Part model, mm, in its own coordinate system. A direction names the side the tool comes from. Coordinates: 2 decimals unless noted, no trailing zeros. Write each loop counter-clockwise with the first axis right and the second up, starting at its lowest first coordinate (ties: lowest second). Pieces come first, ordered by that corner, then holes. Notation, with made-up numbers: (89.25, 12.5) -> (111.25, 12.5) arc R22 cw to (111.25, 47.5) -> close; hole circle Ø11 at (87.25, 13.5). An arc over 180 degrees is marked (long way). Write item = value, one per line. Start each with the question number.
Q1. Band-saw the part on C-C, the plane y = -10.5. List the corners of the cut face in (x, z), plus the area to 3 significant figures.
Q2. Pull direction Z, two halves, no side cores. Call faces 5 (the flat face through (-13, 3, 15.47)), 6 (the flat face through (0, 1, 3)), 7 (the flat face through (-13, 3, 25.4)): released by +Z, released by -Z, zero draft, split by the parting line, or undercut.
Q3. Band-saw the part on D-D, the plane x = -13. List the corners of the cut face in (y, z), plus the area to 3 significant figures.
Q4. Pin check, flat tips, straight feed: P1, Ø5, axis at x = -8, y = -6.5, coming from the +Z side; P2, Ø5, axis at x = -7, z = 3.5, coming from the -Y side. Stop position of each tip, or through.
Q5. Tool access for faces 1 (the flat face through (-20.222, -13, -3)), 2 (the flat face through (-9.744, 3, 12)), 3 (the flat face through (-13, 0, 16)), 4 (the flat face through (-13, 6.35, 6)): list every direction of +Z, -Z, +X, -X, +Y, -Y with a clear straight run to the whole face (end or side of a thin tool).
Q6. Probe line 1 (Z direction, x = -15, y = 1.5); line 2 (Y direction, x = -6.25, z = -5); line 3 (Z direction, x = -3.75, y = -10). List the from-to ranges inside material, lowest first.
Q7. Band-saw the part on B-B, the plane z = 11. List the corners of the cut face in (x, y).
Q8. Band-saw the part on A-A, the plane x = -18.5. List the corners of the cut face in (y, z), plus the area to 3 significant figures.
Autodesk Inventor part; units mm, degrees
ref_plane "YZ Plane" through (0, 0, 0) normal (1, 0, 0) x (0, 1, 0)
ref_plane "XZ Plane" through (0, 0, 0) normal (0, 1, 0) x (-1, 0, 0)
ref_plane "XY Plane" through (0, 0, 0) normal (0, 0, 1) x (1, 0, 0)
sketch "Sketch1" plane through (0, 0, 0) normal (0, 1, 0) x (-1, 0, 0)
  line L0 (0, 0) -> (25.4, 0)
  line L1 (25.4, 0) -> (25.4, 25.4)
  line L2 (25.4, 25.4) -> (0, 25.4)
  line L3 (0, 25.4) -> (0, 0)
  dimension "d0" = 25.4
  dimension "d1" = 25.4
extrude "Extrusion1" add sketch "Sketch1" along normal blind 6.35
sketch "Sketch2" plane through (0, 6.35, 0) normal (0, 1, 0) x (1, 0, 0)
  line L0 (0, 0) -> (-25.4, 0)
  line L1 (0, 0) -> (-25.4, 0)
  line L2 (-25.4, 0) -> (-25.4, 6.35)
  line L3 (-25.4, 6.35) -> (0, 6.35)
  line L4 (0, 6.35) -> (0, 0)
  dimension "d4" = 6.35
extrude "Extrusion2" add sketch "Sketch2" against normal blind 31.75
sketch "Sketch3" plane through (-25.4, 0, 0) normal (0, 0, 1) x (1, 0, 0)
  line L0 (5.1775, -6.7435) -> (19.8333, -6.7435)
  line L1 (19.8333, -6.7435) -> (19.8333, -19.4435)
  line L2 (19.8333, -19.4435) -> (5.1775, -19.4435)
  line L3 (5.1775, -19.4435) -> (5.1775, -6.7435)
  line L4 (5.1775, -6.7435) -> (19.8333, -19.4435) construction
  line L5 (19.8333, -6.7435) -> (5.1775, -19.4435) construction
  point P0 (25.4, 0)
  point P1 (12.5054, -13.0935)
  dimension "d7" = 14.6558
  dimension "d8" = 12.7
extrude "Extrusion3" cut sketch "Sketch3" against normal blind 31.75
sketch "Sketch4" plane through (0, 0, 0) normal (0, -1, 0) x (1, 0, 0)
  line L0 (-15.7889, 15.4698) -> (-9.7437, 15.4698)
  line L1 (-9.7437, 15.4698) -> (-9.7437, 9.4246)
  line L2 (-9.7437, 9.4246) -> (-15.7889, 9.4246)
  line L3 (-15.7889, 9.4246) -> (-15.7889, 15.4698)
  line L4 (-15.7889, 15.4698) -> (-9.7437, 9.4246) construction
  line L5 (-9.7437, 15.4698) -> (-15.7889, 9.4246) construction
  point P0 (0, 0)
  point P1 (-12.7663, 12.4472)
  dimension "d11" = 6.0452
  dimension "d12" = 6.0452
extrude "Extrusion4" cut sketch "Sketch4" against normal blind 25.4
properties part number "l braket w. squares"
Ans:
q1.outline = (-25.4, -6.35) -> (-20.22, -6.35) -> (-20.22, 0) -> (-25.4, 0) -> close; (-5.57, -6.35) -> (0, -6.35) -> (0, 0) -> (-5.57, 0) -> close
q1.area = 68.2 mm2
q2.face_5 = undercut
q2.face_6 = zero draft
q2.face_7 = released by +Z
q3.outline = (-25.4, -6.35) -> (-19.44, -6.35) -> (-19.44, 0) -> (-25.4, 0) -> close; (-6.74, -6.35) -> (6.35, -6.35) -> (6.35, 9.42) -> (0, 9.42) -> (0, 0) -> (-6.74, 0) -> close; (0, 15.47) -> (6.35, 15.47) -> (6.35, 25.4) -> (0, 25.4) -> close
q3.area = 244 mm2
q4.P1 = 0
q4.P2 = 0
q5.face_1 = +Z, -Z
q5.face_2 = +Y, -Y
q5.face_3 = +Z, +X, -X, -Y
q5.face_4 = +Z, -Z, +X, -X, +Y
q6.line_1 = -6.35 to 9.42, 15.47 to 25.4
q6.line_2 = -25.4 to -19.44, -6.74 to 6.35
q6.line_3 = -6.35 to 0
q7.outline = (-25.4, 0) -> (-15.79, 0) -> (-15.79, 6.35) -> (-25.4, 6.35) -> close; (-9.74, 0) -> (0, 0) -> (0, 6.35) -> (-9.74, 6.35) -> close
q8.outline = (-25.4, -6.35) -> (-19.44, -6.35) -> (-19.44, 0) -> (-25.4, 0) -> close; (-6.74, -6.35) -> (6.35, -6.35) -> (6.35, 25.4) -> (0, 25.4) -> (0, 0) -> (-6.74, 0) -> close
q8.area = 282 mm2
